Input: dimensioned drawing with shaded views. Units: mm. Origin: part minimum x, y, z. Round coordinates to 2 decimals unless told otherwise and drop trailing zeros. Order: outer loops, then holes, each group sorted by start corner. A loop starts at its lowest first (then second) coordinate and runs counter-clockwise, first axis right, second up. Notation, with made-up numbers: M -17,-13 L 37,-13 A5 cw 37,-4 Z; hole C 10.25,75 d10. An arc over 180 degrees is marked long. Use one line per item in the form item = value. Start each with the question number.
Q1. Section B-B (x = 50.8). Return the cut outline in (y, z), plus the area to 3 significant figures.
Q2. Section C-C (x = 867.5). Return the cut outline in (y, z).
Q3. Material intervals for probe 1 along X at (y, z) = (356.5, 35); probe 2 along Z at (x, y) = (50.8, 275); probe 3 along Y at (x, z) = (861.5, 36), sorted ascending.
Q4. Contact query for flat-ended pins moving along their axis: pin 1 (1.5 mm diameter, centred on x = 844, z = 10, fed in from -Y); pin 2 (6 mm diameter, centred on x = 438, z = 47.5, fed in from +Y); pin 3 (10 mm diameter, centred on x = 440.5, z = 41, fed in from +Y). Output: stop coordinate, or through.
Q5. Section D-D (x = 285). Return the cut outline in (y, z).
Q6. Section A-A (z = 19.05). Return the cut outline in (x, y).
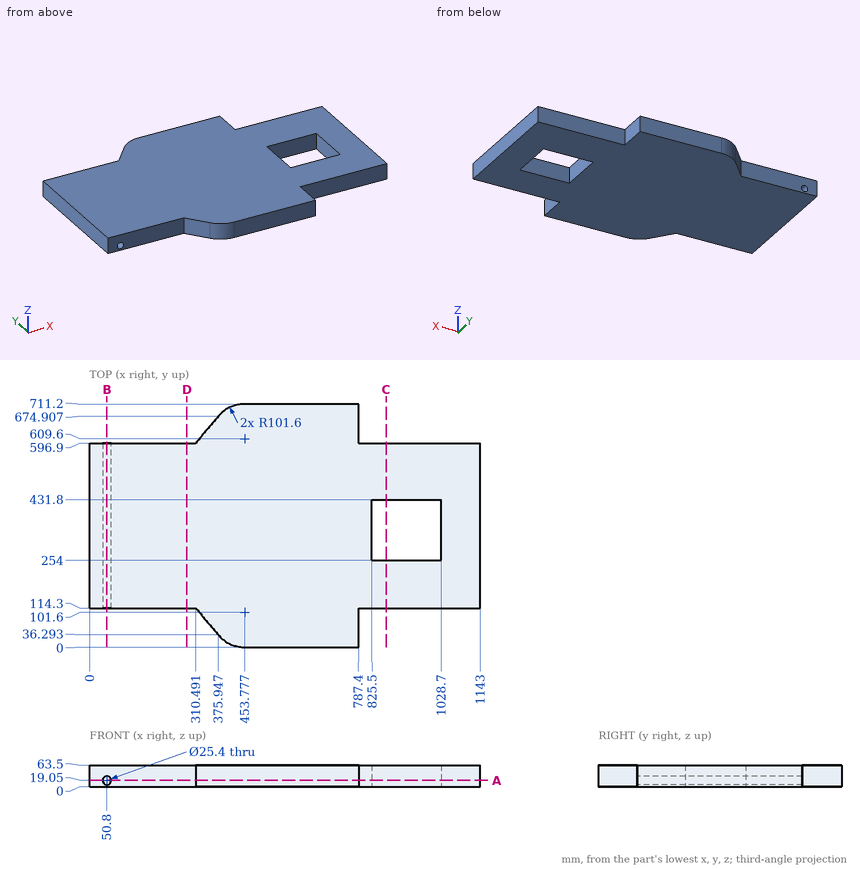
Results list:
q1.outline = M 114.3,0 L 596.9,0 L 596.9,6.35 L 114.3,6.35 Z; M 114.3,31.75 L 596.9,31.75 L 596.9,63.5 L 114.3,63.5 Z
q1.area = 18,400 mm2
q2.outline = M 114.3,0 L 254,0 L 254,63.5 L 114.3,63.5 Z; M 431.8,0 L 596.9,0 L 596.9,63.5 L 431.8,63.5 Z
q3.probe_1 = 0 to 825.5, 1028.7 to 1143
q3.probe_2 = 0 to 6.35, 31.75 to 63.5
q3.probe_3 = 114.3 to 254, 431.8 to 596.9
q4.pin_1 = 114.3
q4.pin_2 = 710.39
q4.pin_3 = 710.86
q5.outline = M 114.3,0 L 596.9,0 L 596.9,63.5 L 114.3,63.5 Z
q6.outline = M 0,114.3 L 38.1,114.3 L 38.1,596.9 L 0,596.9 Z; M 63.5,114.3 L 310.49,114.3 L 375.95,36.29 A101.6 ccw 453.78,0 L 787.4,0 L 787.4,114.3 L 1143,114.3 L 1143,596.9 L 787.4,596.9 L 787.4,711.2 L 453.78,711.2 A101.6 ccw 375.95,674.91 L 310.49,596.9 L 63.5,596.9 Z; hole M 825.5,254 L 1028.7,254 L 1028.7,431.8 L 825.5,431.8 Z
